```python
from build123d import *

# Parameters (mm, degrees)
F0_W     = 50.8
F0_H     = 50.8
F1_DEPTH = 50.8
F2_W     = 38.1
F2_H     = 38.1
F3_DEPTH = 50.8
F4_W     = 38.1
F4_H     = 38.1
F5_DEPTH = 50.8
F6_W     = 38.1
F6_H     = 38.1
F7_DEPTH = 50.8


with BuildPart() as f1:
    # F0 (on Right) → F1 (new body)
    with BuildSketch(Plane.YZ):
        with Locations((-25.4, -25.4)):
            Rectangle(F0_W, F0_H)
    extrude(amount=F1_DEPTH)

    # F2 (on face) → F3 (cut)
    with BuildSketch(Plane.YZ.offset(50.8)):
        with Locations((-25.621607, -25.606393)):
            Rectangle(F2_W, F2_H)
    extrude(amount=-F3_DEPTH, mode=Mode.SUBTRACT)

    # F4 (on face) → F5 (cut)
    with BuildSketch(Plane.XZ.offset(50.8)):
        with Locations((25.222066, -24.840273)):
            Rectangle(F4_W, F4_H)
    extrude(amount=-F5_DEPTH, mode=Mode.SUBTRACT)

    # F6 (on face) → F7 (cut)
    with BuildSketch(Plane.XY):
        with Locations((25.782557, -25.907018)):
            Rectangle(F6_W, F6_H)
    extrude(amount=-F7_DEPTH, mode=Mode.SUBTRACT)


solid = f1.part
```
Input: part model. Units: mm. Frame: model coordinates. A direction names the side the tool comes from. Coordinates: 2 decimals unless noted, no trailing zeros. Order: outer loops, then holes, each group sorted by start corner. A loop starts at its lowest first (then second) coordinate and runs counter-clockwise, first axis right, second up. Notation, with made-up numbers: (21, -22.5) - (40, -22.5) arc R11 ccw to (40, -9.5) - close; hole circle Ø10 at (40.25, 37). An arc over 180 degrees is marked (long way). Put each result on its own line as item: value.
1. Draft query along Y for faces 1 (the face through (27.1, -44.957, -44.1)), 2 (the face through (25, -3, -43.89)), 3 (the face through (25, -50.8, -3)). Return one class per face: pulls with the +Y half, pulls with the -Y half, needs draft (parallel to the pull), parting line crosses it, or undercut.
Report:
face 1: undercut
face 2: needs draft
face 3: pulls with the -Y half
2. Cut plane B-B on x = 23. Return the cut outline in (y, z), then the cut area to 3 significant figures.
Report:
outline: (-50.8, -50.8) - (-44.96, -50.8) - (-44.96, -43.89) - (-50.8, -43.89) - close; (-50.8, -5.79) - (-44.96, -5.79) - (-44.96, 0) - (-50.8, 0) - close; (-6.86, -50.8) - (0, -50.8) - (0, -43.89) - (-6.57, -43.89) - (-6.57, -44.66) - (-6.86, -44.66) - close; (-6.86, -5.79) - (0, -5.79) - (0, 0) - (-6.86, 0) - close
area: 161 mm2
3. Line query: line 1 along Y through (x, z) = (47, -20.5); line 2 along Z through (x, y) = (36.5, -4); line 3 along Z through (x, y) = (2.5, -11.5). Output: solid intervals per line, ascending.
Report:
line 1: y = -50.8 to -44.67, -6.57 to 0
line 2: z = -50.8 to -43.89, -5.79 to 0
line 3: z = -50.8 to -44.66, -6.56 to 0
4. Cut plane D-D on z = -4.5. Return the cut outline in (x, y), then the cut area to 3 significant figures.
Report:
outline: (0, -50.8) - (50.8, -50.8) - (50.8, 0) - (0, 0) - close; hole (6.73, -44.96) - (44.83, -44.96) - (44.83, -6.86) - (6.73, -6.86) - close
area: 1,130 mm2
5. Cut plane A-A on z = -11. Return the cut outline in (x, y), then the cut area to 3 significant figures.
Report:
outline: (0, -50.8) - (6.17, -50.8) - (6.17, -44.67) - (0, -44.67) - close; (0, -6.57) - (6.17, -6.57) - (6.17, 0) - (0, 0) - close; (44.27, -50.8) - (50.8, -50.8) - (50.8, -44.67) - (44.83, -44.67) - (44.83, -44.96) - (44.27, -44.96) - close; (44.27, -6.57) - (50.8, -6.57) - (50.8, 0) - (44.27, 0) - close
area: 161 mm2
6. Cut plane C-C on y = -3.5. Return the cut outline in (x, z), then the cut area to 3 significant figures.
Report:
outline: (0, -50.8) - (50.8, -50.8) - (50.8, 0) - (0, 0) - close; hole (6.17, -43.89) - (44.27, -43.89) - (44.27, -5.79) - (6.17, -5.79) - close
area: 1,130 mm2
7. Reachability of faces 4 (the face through (44.272, -48, -25)), 5 (the face through (48, -26, -6.556)), 6 (the face through (26, -6.857, -48)) from +Z, -Z, +X, -X, +Y, -Y: full face, straight path, thin tool, end or side. Return the list, or none.
Report:
face 4: +Y, -Y
face 5: +X, -X
face 6: +Z, -Z
